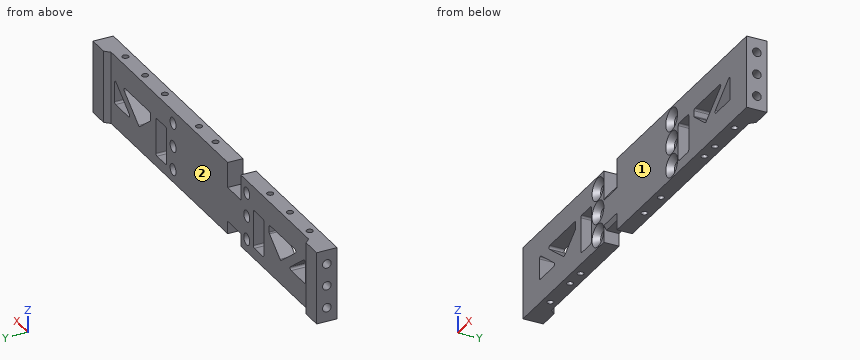
```python
from build123d import *
from OCP.BRepFilletAPI import BRepFilletAPI_MakeChamfer

# Parameters (mm, degrees)
ESBO_O1_W                                           = 340
ESBO_O1_H                                           = 57
RESSALTO_EXTRUS_O1_DEPTH                            = 12
ESBO_O2_W                                           = 20
ESBO_O2_H                                           = 57
RESSALTO_EXTRUS_O2_DEPTH                            = 4
BROCA_DE_ROSQUEAR_PARA_TARRAXA_DE_M81_D             = 6.8
BROCA_DE_ROSQUEAR_PARA_TARRAXA_DE_M81_DEPTH         = 15
BROCA_DE_ROSQUEAR_PARA_TARRAXA_DE_M81_TIP           = 2.042926105
BROCA_DE_ROSQUEAR_PARA_TARRAXA_DE_M82_D             = 6.8
BROCA_DE_ROSQUEAR_PARA_TARRAXA_DE_M82_DEPTH         = 15
BROCA_DE_ROSQUEAR_PARA_TARRAXA_DE_M82_TIP           = 2.042926105
ESBO_O7_W                                           = 20
ESBO_O7_H                                           = 10
ESBO_O7_H_2                                         = 20
CORTE_EXTRUS_O1_DEPTH                               = 345.953620071
CHANFRO1_SIZE                                       = 2
CHANFRO1_SIZE2                                      = 3.464101615
CHANFRO3_SIZE                                       = 4
BROCA_DE_ROSQUEAR_PARA_TARRAXA_DE_M61_D             = 5
BROCA_DE_ROSQUEAR_PARA_TARRAXA_DE_M61_DEPTH         = 15
BROCA_DE_ROSQUEAR_PARA_TARRAXA_DE_M61_TIP           = 1.502151548
BROCA_DE_ROSQUEAR_PARA_TARRAXA_DE_M62_D             = 5
BROCA_DE_ROSQUEAR_PARA_TARRAXA_DE_M62_DEPTH         = 15
BROCA_DE_ROSQUEAR_PARA_TARRAXA_DE_M62_TIP           = 1.502151548
ESCAREADO_PARA_PARAFUSO_ALLEN_SEXTAVADO_D           = 9
ESCAREADO_PARA_PARAFUSO_ALLEN_SEXTAVADO_DEPTH       = 15
ESCAREADO_PARA_PARAFUSO_ALLEN_SEXTAVADO_CSINK_D     = 17.92
ESCAREADO_PARA_PARAFUSO_ALLEN_SEXTAVADO_CSINK_ANGLE = 90
ESCAREADO_PARA_PARAFUSO_ALLEN_SEXTAVADO_TIP         = 2.703872786
ESBO_O19_W                                          = 16
ESBO_O19_H                                          = 30
CORTE_EXTRUS_O3_DEPTH                               = 346.115922554
FILETE6_R                                           = 1.5


with BuildPart() as part:
    # Esboço1 → Ressalto-extrusão1 (new body)
    with BuildSketch(Plane(origin=(0, 0, 0), x_dir=(1, 0, 0), z_dir=(0, 1, 0))):
        with Locations((170, 28.5)):
            Rectangle(ESBO_O1_W, ESBO_O1_H)
    extrude(amount=RESSALTO_EXTRUS_O1_DEPTH)

    # Esboço2 → Ressalto-extrusão2 (add)
    with BuildSketch(Plane(origin=(0, 12, 0), x_dir=(1, 0, 0), z_dir=(0, 1, 0))):
        with Locations((10, 28.5)):
            Rectangle(ESBO_O2_W, ESBO_O2_H)
        with Locations((330, 28.5)):
            Rectangle(ESBO_O2_W, ESBO_O2_H)
    extrude(amount=RESSALTO_EXTRUS_O2_DEPTH)

    # Broca de rosquear para tarraxa de M81
    with Locations(Plane.ZY):
        with Locations((-46, 8), (-28.5, 8), (-11, 8)):
            Hole(BROCA_DE_ROSQUEAR_PARA_TARRAXA_DE_M81_D / 2, depth=BROCA_DE_ROSQUEAR_PARA_TARRAXA_DE_M81_DEPTH)
            with Locations((0, 0, -(BROCA_DE_ROSQUEAR_PARA_TARRAXA_DE_M81_DEPTH + BROCA_DE_ROSQUEAR_PARA_TARRAXA_DE_M81_TIP / 2))):  # 118° drill point
                Cone(0, BROCA_DE_ROSQUEAR_PARA_TARRAXA_DE_M81_D / 2, BROCA_DE_ROSQUEAR_PARA_TARRAXA_DE_M81_TIP, mode=Mode.SUBTRACT)

    # Broca de rosquear para tarraxa de M82
    with Locations(Plane(origin=(340, 0, 0), x_dir=(0, 0, -1), z_dir=(1, 0, 0))):
        with Locations((28.5, 8), (11, 8), (46, 8)):
            Hole(BROCA_DE_ROSQUEAR_PARA_TARRAXA_DE_M82_D / 2, depth=BROCA_DE_ROSQUEAR_PARA_TARRAXA_DE_M82_DEPTH)
            with Locations((0, 0, -(BROCA_DE_ROSQUEAR_PARA_TARRAXA_DE_M82_DEPTH + BROCA_DE_ROSQUEAR_PARA_TARRAXA_DE_M82_TIP / 2))):  # 118° drill point
                Cone(0, BROCA_DE_ROSQUEAR_PARA_TARRAXA_DE_M82_D / 2, BROCA_DE_ROSQUEAR_PARA_TARRAXA_DE_M82_TIP, mode=Mode.SUBTRACT)

    # Esboço7 → Corte-extrusão1 (cut, through all)
    with BuildSketch(Plane(origin=(0, 12, 0), x_dir=(1, 0, 0), z_dir=(0, 1, 0))):
        with Locations((133, 52)):
            Rectangle(ESBO_O7_W, ESBO_O7_H)
        with Locations((133, 10)):
            Rectangle(ESBO_O7_W, ESBO_O7_H_2)
    extrude(amount=-CORTE_EXTRUS_O1_DEPTH, mode=Mode.SUBTRACT)

    # Chanfro1: one chamfer whose edges measure the first distance from different faces: ONE call of the kernel's chamfer builder (chamfer() names one face for all edges)
    chanfro1_edges_1 = [part.edges().sort_by_distance(p)[0] for p in [
        (133, 0, -47),
    ]]
    chanfro1_side_1 = [part.faces().sort_by_distance(p)[0] for p in [
        (133, 6, -47),
    ]]
    chanfro1_edges_2 = [part.edges().sort_by_distance(p)[0] for p in [
        (133, 0, -20),
    ]]
    chanfro1_side_2 = [part.faces().sort_by_distance(p)[0] for p in [
        (133, 6, -20),
    ]]
    chanfro1 = BRepFilletAPI_MakeChamfer(part.part.solid().wrapped)
    for e in chanfro1_edges_1:
        chanfro1.Add(CHANFRO1_SIZE, CHANFRO1_SIZE2, e.wrapped, chanfro1_side_1[0].wrapped)  # the first distance lies on this face
    for e in chanfro1_edges_2:
        chanfro1.Add(CHANFRO1_SIZE, CHANFRO1_SIZE2, e.wrapped, chanfro1_side_2[0].wrapped)  # the first distance lies on this face
    add(Compound.cast(chanfro1.Shape()), mode=Mode.REPLACE)

    # Chanfro3
    chanfro3_edges = [part.edges().sort_by_distance(p)[0] for p in [
        (20, 16, -28.5),
        (320, 16, -28.5),
    ]]
    chamfer(chanfro3_edges, length=CHANFRO3_SIZE - 0.0001)  # a hair under: the kernel refuses the full size

    # Broca de rosquear para tarraxa de M61
    with Locations(Plane(origin=(0, 0, -57), x_dir=(-1, 0, 0), z_dir=(0, 0, -1))):
        with Locations((-310, 6), (-280, 6), (-30, 6), (-60, 6), (-264, 6), (-76, 6), (-198, 6), (-173, 6)):
            Hole(BROCA_DE_ROSQUEAR_PARA_TARRAXA_DE_M61_D / 2, depth=BROCA_DE_ROSQUEAR_PARA_TARRAXA_DE_M61_DEPTH)
            with Locations((0, 0, -(BROCA_DE_ROSQUEAR_PARA_TARRAXA_DE_M61_DEPTH + BROCA_DE_ROSQUEAR_PARA_TARRAXA_DE_M61_TIP / 2))):  # 118° drill point
                Cone(0, BROCA_DE_ROSQUEAR_PARA_TARRAXA_DE_M61_D / 2, BROCA_DE_ROSQUEAR_PARA_TARRAXA_DE_M61_TIP, mode=Mode.SUBTRACT)

    # Broca de rosquear para tarraxa de M62
    with Locations(Plane.XY):
        with Locations((30, 6), (60, 6), (280, 6), (310, 6), (90, 6), (250, 6), (173, 6), (198, 6)):
            Hole(BROCA_DE_ROSQUEAR_PARA_TARRAXA_DE_M62_D / 2, depth=BROCA_DE_ROSQUEAR_PARA_TARRAXA_DE_M62_DEPTH)
            with Locations((0, 0, -(BROCA_DE_ROSQUEAR_PARA_TARRAXA_DE_M62_DEPTH + BROCA_DE_ROSQUEAR_PARA_TARRAXA_DE_M62_TIP / 2))):  # 118° drill point
                Cone(0, BROCA_DE_ROSQUEAR_PARA_TARRAXA_DE_M62_D / 2, BROCA_DE_ROSQUEAR_PARA_TARRAXA_DE_M62_TIP, mode=Mode.SUBTRACT)

    # Escareado para parafuso Allen sextavado escareado de M82
    with Locations(Plane(origin=(0, 0, 0), x_dir=(-1, 0, 0), z_dir=(0, -1, 0))):
        with Locations((-114, 47), (-114, 28.5), (-114, 10), (-226, 47), (-226, 28.5), (-226, 10)):
            CounterSinkHole(ESCAREADO_PARA_PARAFUSO_ALLEN_SEXTAVADO_D / 2, ESCAREADO_PARA_PARAFUSO_ALLEN_SEXTAVADO_CSINK_D / 2, depth=ESCAREADO_PARA_PARAFUSO_ALLEN_SEXTAVADO_DEPTH, counter_sink_angle=ESCAREADO_PARA_PARAFUSO_ALLEN_SEXTAVADO_CSINK_ANGLE)
            with Locations((0, 0, -(ESCAREADO_PARA_PARAFUSO_ALLEN_SEXTAVADO_DEPTH + ESCAREADO_PARA_PARAFUSO_ALLEN_SEXTAVADO_TIP / 2))):  # 118° drill point
                Cone(0, ESCAREADO_PARA_PARAFUSO_ALLEN_SEXTAVADO_D / 2, ESCAREADO_PARA_PARAFUSO_ALLEN_SEXTAVADO_TIP, mode=Mode.SUBTRACT)

    # Esboço19 → Corte-extrusão3 (cut, through all)
    with BuildSketch(Plane.XZ):
        Polygon((25, -18.5), (25, -38.5), (51, -38.5), align=None)
        Polygon((36.480853627, -18.5), (62.480853627, -38.5), (80, -25.023733559), (80, -18.5), (62.480853627, -18.5), align=None)
        with Locations((96, -33.5)):
            Rectangle(ESBO_O19_W, ESBO_O19_H)
        with Locations((244, -33.5)):
            Rectangle(ESBO_O19_W, ESBO_O19_H)
        Polygon((260, -25.023733559), (260, -18.5), (277.519146373, -18.5), (303.519146373, -18.5), (277.519146373, -38.5), align=None)
        Polygon((315, -38.5), (289, -38.5), (315, -18.5), align=None)
    extrude(amount=-CORTE_EXTRUS_O3_DEPTH, mode=Mode.SUBTRACT)

    # Filete6
    filete6_edges = [part.edges().sort_by_distance(p)[0] for p in [
        (36.480853627, 6, -18.5),
        (80, 6, -18.5),
        (80, 6, -25.023733559),
        (62.480853627, 6, -38.5),
        (104, 6, -48.5),
        (88, 6, -48.5),
        (88, 6, -18.5),
        (104, 6, -18.5),
        (252, 6, -18.5),
        (252, 6, -48.5),
        (236, 6, -48.5),
        (236, 6, -18.5),
        (277.519146373, 6, -38.5),
        (260, 6, -25.023733559),
        (260, 6, -18.5),
        (303.519146373, 6, -18.5),
        (315, 6, -18.5),
        (315, 6, -38.5),
        (289, 6, -38.5),
        (25, 6, -18.5),
        (51, 6, -38.5),
        (25, 6, -38.5),
    ]]
    fillet(filete6_edges, radius=FILETE6_R)


solid = part.part
```
Read the model definition and answer for the solid it produces. Units are mm, in the model's axes. Face numbers are marked on the shaded views. Round coordinates to 2 decimals unless told otherwise and drop trailing zeros. Write each loop counter-clockwise with the first axis right and the second up, starting at its lowest first coordinate (ties: lowest second). Pieces come first, ordered by that corner, then holes. Notation, with made-up numbers: (-2.5, -24) - (10.5, -24) arc R22 ccw to (10.5, 6) - close; hole circle Ø5 at (-29.75, -13.75). An arc over 180 degrees is marked (long way). One line per item, written item: value.
Q1. For a pull along X with two mould halves and no side action, classify the marked faces 1 and 2 as pulls with the +X half, pulls with the -X half, needs draft (parallel to the pull), parting line crosses it, or undercut.
The answers:
face 1: needs draft
face 2: undercut
Q2. Find section B-B (x = 53.5). Determine the outline of the cut face in (y, z).
The answers:
outline: (0, -57) - (12, -57) - (12, -31.59) - (0, -31.59) - close; (0, -18.5) - (12, -18.5) - (12, 0) - (0, 0) - close
Q3. Find section A-A (x = 226). Determine the outline of the cut face in (y, z).
The answers:
outline: (0, -57) - (12, -57) - (12, -51.5) - (4.46, -51.5) - (0, -55.96) - close; (0, -38.04) - (4.46, -42.5) - (12, -42.5) - (12, -33) - (4.46, -33) - (0, -37.46) - close; (0, -19.54) - (4.46, -24) - (12, -24) - (12, -14.5) - (4.46, -14.5) - (0, -18.96) - close; (0, -1.04) - (4.46, -5.5) - (12, -5.5) - (12, 0) - (0, 0) - close
Q4. Each of these flat-tipped pins is pushed along its axis until it touches: P1, Ø3, axis at x = 60, y = 6, coming from the -Z side; P2, Ø3, axis at x = 173, y = 6, coming from the +Z side; P3, Ø1.5, axis at x = 36, z = -26, coming from the +Y side. Where does it stop, or does it pass through?
The answers:
P1: stops at z = -41.4
P2: stops at z = -15.6
P3: stops at y = 12
Q5. Straight lines are drawn through the part: line 1 (X direction, y = 11.75, z = -39.5); line 2 (Z direction, x = 114, y = 7.25); line 3 (Y direction, x = 264, z = -47.25). For each, find the intervals that lie inside material, in ascending order. Write a range as from..to.
The answers:
line 1: x = 0..88, 104..236, 252..340
line 2: z = -57..-51.5, -42.5..-33, -24..-14.5, -5.5..0
line 3: y = 0..3.5, 8.5..12
